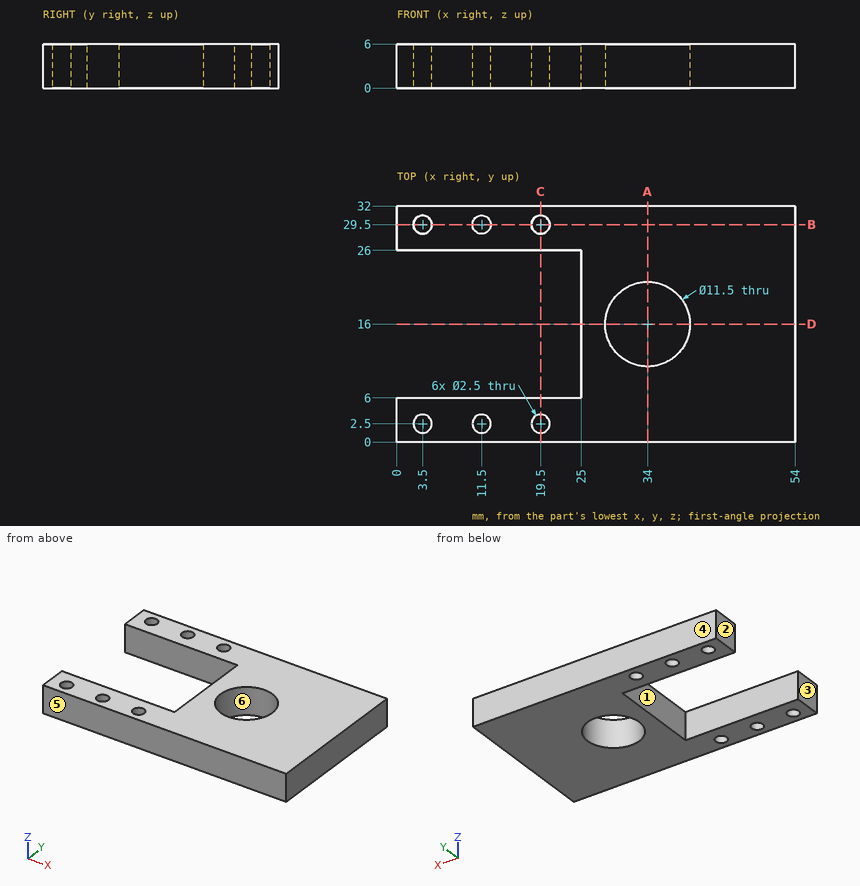
Print and shaded views of the part. All mm, measured from the part's lowest x, y and z. A direction names the side the tool comes from. Give positions to 0.01 mm unless a question says otherwise; leave off trailing zeros. Order: outer loops, then holes, each group sorted by start corner. A loop starts at its lowest first (then second) coordinate and runs counter-clockwise, first axis right, second up. Notation, with made-up numbers: (21.5, 59.5) - (48.5, 59.5) arc R6 ccw to (48.5, 66.5) - close; hole circle Ø7 at (57.25, -28.5). An arc over 180 degrees is marked (long way). One line per item, written item: value.
Item 1: Slice it at C-C (x = 19.5). List the corners of the cut face in (y, z).
Response values:
outline: (0, 0) - (1.25, 0) - (1.25, 6) - (0, 6) - close; (3.75, 0) - (6, 0) - (6, 6) - (3.75, 6) - close; (26, 0) - (28.25, 0) - (28.25, 6) - (26, 6) - close; (30.75, 0) - (32, 0) - (32, 6) - (30.75, 6) - close
Item 2: Slice it at D-D (y = 16). List the corners of the cut face in (x, z), then the cut area to 3 significant figures.
Response values:
outline: (25, 0) - (28.25, 0) - (28.25, 6) - (25, 6) - close; (39.75, 0) - (54, 0) - (54, 6) - (39.75, 6) - close
area: 105 mm2
Item 3: Tool access for the marked faces 1 and 2: list every direction of +Z, -Z, +X, -X, +Y, -Y with a clear straight run to the whole face (end or side of a thin tool).
Response values:
face 1: +Z, -Z, -X
face 2: +Z, -Z, -X, +Y, -Y
Item 4: Slice it at A-A (x = 34). List the corners of the cut face in (y, z), then the cut area to 3 significant figures.
Response values:
outline: (0, 0) - (10.25, 0) - (10.25, 6) - (0, 6) - close; (21.75, 0) - (32, 0) - (32, 6) - (21.75, 6) - close
area: 123 mm2
Item 5: Pin check, flat tip, straight feed: pin 1 Ø3 at (y, z) = (18, 4.5) entering from -X. Stop position of the tip, or through.
Response values:
pin 1: x = 25
Item 6: Slice it at B-B (y = 29.5). List the corners of the cut face in (x, z).
Response values:
outline: (0, 0) - (2.25, 0) - (2.25, 6) - (0, 6) - close; (4.75, 0) - (10.25, 0) - (10.25, 6) - (4.75, 6) - close; (12.75, 0) - (18.25, 0) - (18.25, 6) - (12.75, 6) - close; (20.75, 0) - (54, 0) - (54, 6) - (20.75, 6) - close
Item 7: Wall check: line 1 (X direction, y = 29.5, z = 4.35); line 2 (Y direction, x = 18, z = 3); line 3 (Y direction, x = 2.5, z = 2.6). Give the ranges that are in metal, low to high.
Response values:
line 1: 0 to 2.25, 4.75 to 10.25, 12.75 to 18.25, 20.75 to 54
line 2: 0 to 6, 26 to 32
line 3: 0 to 1.75, 3.25 to 6, 26 to 28.75, 30.25 to 32
Item 8: Two-plate mould, pull along Y, no slides. Class the marked faces 3, 4, 5 and 6: released by +Y, released by -Y, zero draft, split by the parting line, or undercut.
Response values:
face 3: zero draft
face 4: released by +Y
face 5: released by -Y
face 6: undercut
